Print and shaded views of the part. All mm, measured from the part's lowest x, y and z. A direction names the side the tool comes from. Round coordinates to 2 decimals unless told otherwise and drop trailing zeros. Loops run counter-clockwise (first coordinate to the right, second up) from the corner with the lowest first, then second, coordinate; pieces in that order, holes last. Notation, with made-up numbers: (7.25, -7) - (14.25, -7) arc R28 cw to (14.25, 16) - close; hole circle Ø5 at (20.25, 70.25). An arc over 180 degrees is marked (long way). Use one line per item in the form item = value. Start each with the question number.
Q1. Mould opens along X. For the marked faces 4, 5, 6 and 7 say: released by +X, released by -X, zero draft, split by the parting line, or undercut.
Q2. 3-axis set-ups, long thin cutter, end or side, ignore diameter. For the marked faces 1, 2 and 3: which of +Z, -Z, +X, -X, +Y, -Y reach the whole face in a straight line?
Q3. Saw through at D-D (z = 5). Give the cut face in (x, y), then the cut area to 3 significant figures.
Q4. Saw through at A-A (x = 16.25). Give the cut face in (y, z).
Q5. Pin check, flat tips, straight feed: pin 1 (5 mm diameter, centred on x = 13.5, y = 3, fed in from +Z); pin 2 (2 mm diameter, centred on x = 5, z = 12.5, fed in from +Y); pin 3 (1.2 mm diameter, centred on x = 1, y = 1.5, fed in from +Z). Stop position of each tip, or through.
Q6. Drill centre lines: line 1 (X direction, y = 2.85, z = 5); line 2 (Z direction, x = 15.5, y = 2.1); line 3 (X direction, y = 6.25, z = 7). Where is each one in solid material? Low to high.
Q7. Saw through at C-C (y = 13). Give the cut face in (x, z).
Q8. Saw through at B-B (z = 14.75). Give the cut face in (x, y), then the cut area to 3 significant figures.
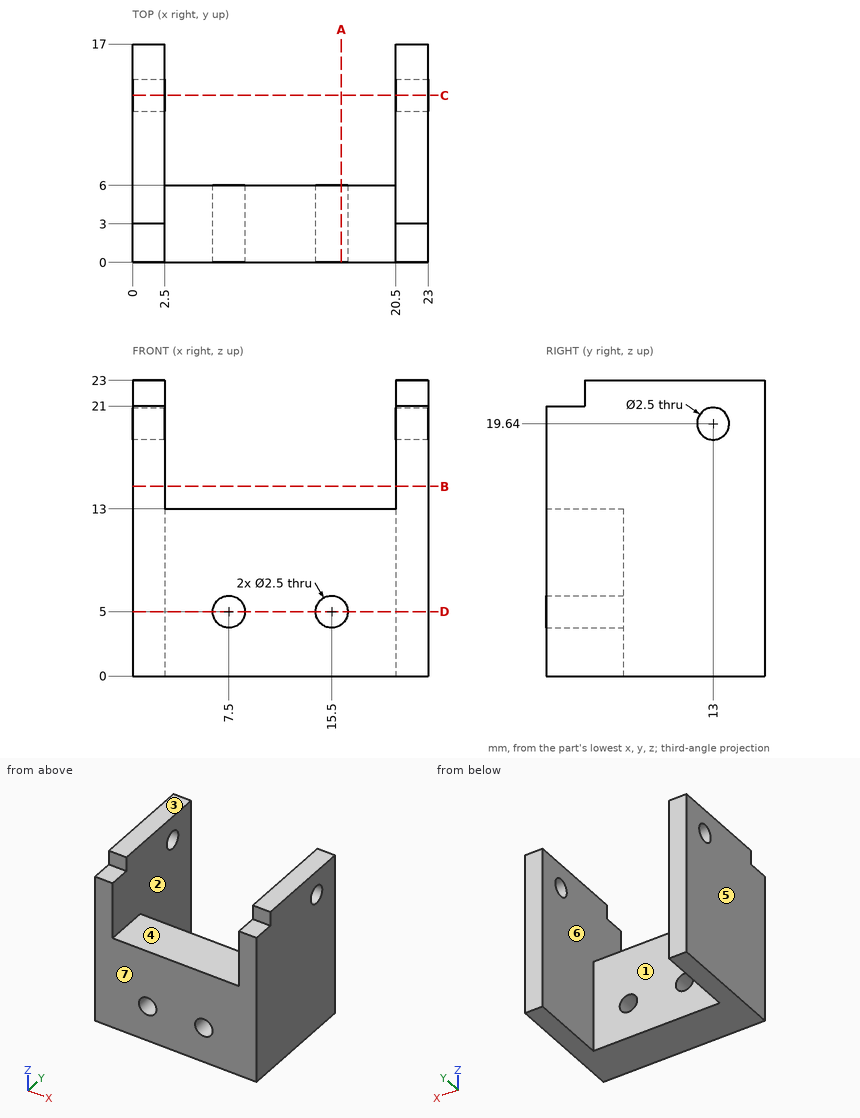
Report:
q1.face_4 = undercut
q1.face_5 = released by -X
q1.face_6 = undercut
q1.face_7 = zero draft
q2.face_1 = +Z, -Z, +Y
q2.face_2 = +Z, +Y
q2.face_3 = +Z, +X, -X, +Y, -Y
q3.outline = (0, 0) - (6.25, 0) - (6.25, 6) - (2.5, 6) - (2.5, 17) - (0, 17) - close; (8.75, 0) - (14.25, 0) - (14.25, 6) - (8.75, 6) - close; (16.75, 0) - (23, 0) - (23, 17) - (20.5, 17) - (20.5, 6) - (16.75, 6) - close
q3.area = 163 mm²
q4.outline = (0, 0) - (6, 0) - (6, 4) - (0, 4) - close; (0, 6) - (6, 6) - (6, 13) - (0, 13) - close
q5.pin_1 = 13
q5.pin_2 = 6
q5.pin_3 = 21
q6.line_1 = 0 to 6.25, 8.75 to 14.25, 16.75 to 23
q6.line_2 = 0 to 3.75, 6.25 to 13
q6.line_3 = 0 to 2.5, 20.5 to 23
q7.outline = (0, 0) - (2.5, 0) - (2.5, 18.39) - (0, 18.39) - close; (0, 20.89) - (2.5, 20.89) - (2.5, 23) - (0, 23) - close; (20.5, 0) - (23, 0) - (23, 18.39) - (20.5, 18.39) - close; (20.5, 20.89) - (23, 20.89) - (23, 23) - (20.5, 23) - close
q8.outline = (0, 0) - (2.5, 0) - (2.5, 17) - (0, 17) - close; (20.5, 0) - (23, 0) - (23, 17) - (20.5, 17) - close
q8.area = 85.0 mm²
